Verification items for the finished model (mm, model axes). Face numbers are marked on the shaded views. Round coordinates to 2 decimals unless told otherwise and drop trailing zeros. Write each loop counter-clockwise with the first axis right and the second up, starting at its lowest first coordinate (ties: lowest second). Pieces come first, ordered by that corner, then holes. Notation, with made-up numbers: M -23.75,49 L -9.75,49 A15 cw -9.75,73 Z; hole C -12,-38.5 d2. An arc over 180 degrees is marked long. One line per question, with ' | ' between items. Start each with the question number.
Q1. Cross-section at D-D (x = -8). Record the boundary of the cut face in (y, z), then the cut area to 3 significant figures.
Q2. Thickness scan on line 1 along Y through (x, z) = (0, 1.2); line 2 along Y through (x, z) = (0.5, 3.2); line 3 along X through (y, z) = (-8.5, 0.3). Record the ranges inside material, lowest first. Write a range as from..to.
Q3. Release check for a two-part mould opening along Y. For the marked faces 1 and 2 record: released by +Y, released by -Y, zero draft, split by the parting line, or undercut.
Q4. Cross-section at B-B (z = 3.1). Record the boundary of the cut face in (x, y).
Q5. Cross-section at A-A (x = 0). Record the boundary of the cut face in (y, z).
Q6. Gauge pin test, flat ends, axial feed: pin 1 (7.5 mm diameter, centred on x = 0, y = -11, fed in from +Z); pin 2 (2 mm diameter, centred on x = -8, z = 1, fed in from +Y). Record the tip position at first contact, or that the pin passes through.
Q7. Cross-section at C-C (y = -19). Record the boundary of the cut face in (x, z).
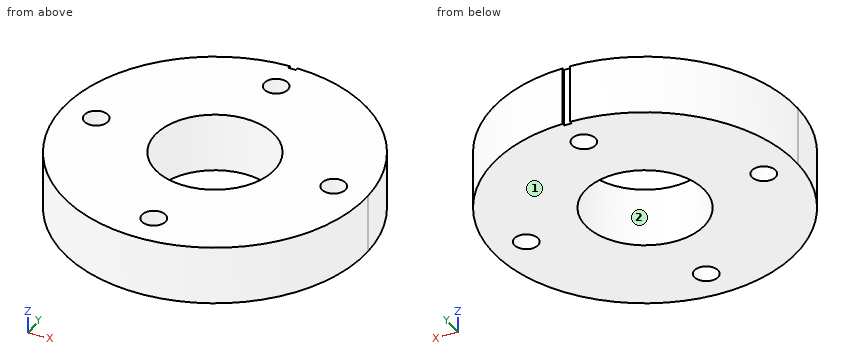
from build123d import *

# Parameters (mm, degrees)
BOSS_EXTRUDE1_DEPTH = 4


with BuildPart() as part:
    # Sketch2 → Boss-Extrude1 (new body)
    with BuildSketch(Plane.XY):
        with BuildLine():
            Line((-0.25, -0.9), (-0.25, -0.703034428))
            ThreePointArc((-0.25, -0.703034428), (-7.371058269, -3.805731448), (-10.3, -11))
            ThreePointArc((-10.3, -11), (0, -21.3), (10.3, -11))
            ThreePointArc((10.3, -11), (7.371058269, -3.805731448), (0.25, -0.703034428))
            Line((0.25, -0.703034428), (0.25, -0.9))
            Line((0.25, -0.9), (-0.25, -0.9))
        make_face()
        with BuildLine():
            ThreePointArc((-8.8, -11), (-8, -11.8), (-7.2, -11))
            ThreePointArc((-7.2, -11), (-8, -10.2), (-8.8, -11))
        make_face(mode=Mode.SUBTRACT)
        with BuildLine():
            ThreePointArc((0.8, -3), (0, -2.2), (-0.8, -3))
            ThreePointArc((-0.8, -3), (0, -3.8), (0.8, -3))
        make_face(mode=Mode.SUBTRACT)
        with BuildLine():
            ThreePointArc((0.8, -19), (0, -18.2), (-0.8, -19))
            ThreePointArc((-0.8, -19), (0, -19.8), (0.8, -19))
        make_face(mode=Mode.SUBTRACT)
        with BuildLine():
            ThreePointArc((8.8, -11), (8, -10.2), (7.2, -11))
            ThreePointArc((7.2, -11), (8, -11.8), (8.8, -11))
        make_face(mode=Mode.SUBTRACT)
        with BuildLine():
            ThreePointArc((4.05, -11), (0, -6.95), (-4.05, -11))
            ThreePointArc((-4.05, -11), (0, -15.05), (4.05, -11))
        make_face(mode=Mode.SUBTRACT)
    extrude(amount=BOSS_EXTRUDE1_DEPTH)


solid = part.part
Determined:
1) outline: M -17.49,0 L -11.8,0 L -11.8,4 L -17.49,4 Z; M -10.2,0 L -4.51,0 L -4.51,4 L -10.2,4 Z | area: 45.5 mm²
2) line 1: y = -21.3..-19.8, -18.2..-15.05, -6.95..-3.8, -2.2..-0.9 | line 2: y = -21.29..-19.62, -18.38..-15.02, -6.98..-3.62, -2.38..-0.71 | line 3: x = -9.99..-3.19, 3.19..9.99
3) face 1: zero draft | face 2: undercut
4) outline: M -0.25,-0.9 L -0.25,-0.7 A10.3 ccw long 0.25,-0.7 L 0.25,-0.9 Z; hole C -8,-11 d1.6; hole C 0,-11 d8.1; hole C 0,-19 d1.6; hole C 0,-3 d1.6; hole C 8,-11 d1.6
5) outline: M -21.3,0 L -19.8,0 L -19.8,4 L -21.3,4 Z; M -18.2,0 L -15.05,0 L -15.05,4 L -18.2,4 Z; M -6.95,0 L -3.8,0 L -3.8,4 L -6.95,4 Z; M -2.2,0 L -0.9,0 L -0.9,4 L -2.2,4 Z
6) pin 1: passes through | pin 2: stops at y = -3.44
7) outline: M -6.49,0 L -0.8,0 L -0.8,4 L -6.49,4 Z; M 0.8,0 L 6.49,0 L 6.49,4 L 0.8,4 Z
